Can you work these out from the drawing? Everything is in mm from the part's minimum corner. A direction names the side the tool comes from. Coordinates: 2 decimals unless noted, no trailing zeros. Write each loop counter-clockwise with the first axis right and the second up, starting at its lowest first coordinate (ties: lowest second). Pieces come first, ordered by that corner, then holes.
(1) Imagine slicing it at D-D, the plane z = 16. List the corners of the cut face in (x, y) for me.
(2) Imagine slicing it at B-B, the plane x = 21.15. List the corners of the cut face in (y, z) for me.
(3) Imagine slicing it at A-A, the plane y = 55. List the corners of the cut face in (x, z) for me, plus the area to 3 significant figures.
(4) For pin 1 Ø1.5 at (x, z) = (15, 17) entering from -Y; pin 2 Ø6.5 at (x, z) = (26.5, 22.5) entering from -Y; pin 3 Ø5 at (x, z) = (8.5, 28) entering from -Y; pin 4 Ø4 at (y, z) = (21, 30) entering from -X, each with a flat end and sliding along its axis, tell me the tip position at first contact or that it passes through.
(5) Please list where these lines run through material, in increasing order: probe 1 along Y at (x, z) = (17, 7); probe 2 along Y at (x, z) = (13.5, 22); probe 3 along Z at (x, y) = (2.5, 26.5).
(6) Which directions (+Z, -Z, +X, -X, +Y, -Y) give clear straight access to the entire face, cutting with the end or side of a thin tool? Please do the marked faces 1 and 2.
(7) Imagine slicing it at C-C, the plane z = 21.15. List the corners of the cut face in (x, y) for me.
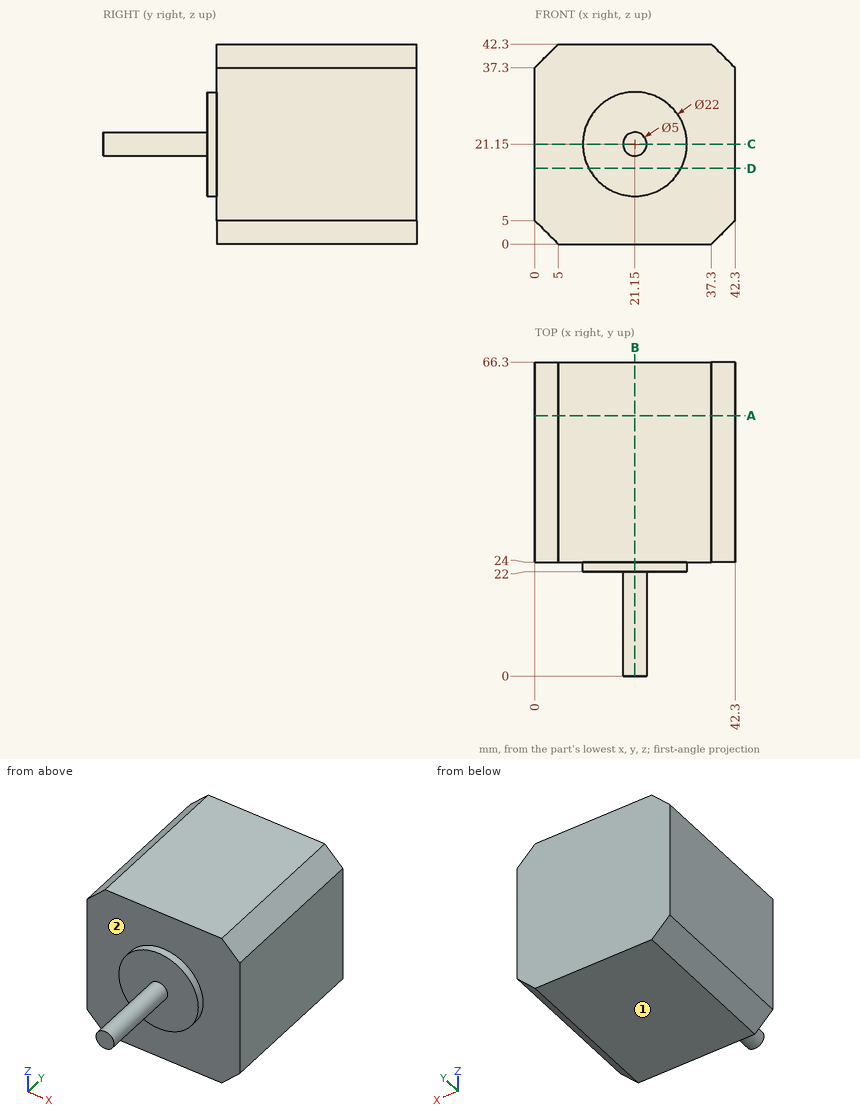
Recorded:
1. outline: (0, 24) - (11.43, 24) - (11.43, 22) - (30.87, 22) - (30.87, 24) - (42.3, 24) - (42.3, 66.3) - (0, 66.3) - close
2. outline: (0, 18.65) - (22, 18.65) - (22, 10.15) - (24, 10.15) - (24, 0) - (66.3, 0) - (66.3, 42.3) - (24, 42.3) - (24, 32.15) - (22, 32.15) - (22, 23.65) - (0, 23.65) - close
3. outline: (0, 5) - (5, 0) - (37.3, 0) - (42.3, 5) - (42.3, 37.3) - (37.3, 42.3) - (5, 42.3) - (0, 37.3) - close
3. area: 1,740 mm2
4. pin 1: stops at y = 22
4. pin 2: stops at y = 0
4. pin 3: stops at y = 24
4. pin 4: stops at x = 12.76
5. probe 1: y = 24 to 66.3
5. probe 2: y = 22 to 66.3
5. probe 3: z = 2.5 to 39.8
6. face 1: -Z, +X, -X, +Y, -Y
6. face 2: -Y
7. outline: (0, 24) - (10.15, 24) - (10.15, 22) - (18.65, 22) - (18.65, 0) - (23.65, 0) - (23.65, 22) - (32.15, 22) - (32.15, 24) - (42.3, 24) - (42.3, 66.3) - (0, 66.3) - close
